Geometry: final body of the model. Coordinates: model frame, mm. A direction names the side the tool comes from. Round coordinates to 2 decimals unless told otherwise and drop trailing zeros. Loops run counter-clockwise (first coordinate to the right, second up) from the corner with the lowest first, then second, coordinate; pieces in that order, holes last. Notation, with made-up numbers: (-14, 38) - (32, 38) arc R5 ccw to (32, 47) - close; hole circle Ø3 at (10, 19.5). An arc over 180 degrees is marked (long way). Answer in a Markdown table with one row per item. Add a question column.
from build123d import *

# Parameters (mm, degrees)
CUT_EXTRUDE1_DEPTH      = 74.786855198
CUT_EXTRUDE1_DEPTH_BACK = 74.786855198
SKETCH3_W               = 2
SKETCH3_H               = 17
CUT_EXTRUDE2_DEPTH      = 44
CIRPATTERN1_COUNT       = 3


with BuildPart() as part:
    # Sketch1 → Revolve1 (revolve)
    with BuildSketch(Plane.XY, mode=Mode.PRIVATE) as revolve1_sk:
        Polygon((8, 0), (11.5, 0), (11.5, 19), (10, 19), (10, 46), (12.5, 46), (16.5, 70), (8, 70), align=None)
    revolve(revolve1_sk.sketch.rotate(Axis((0, 72.635796235, 0), (0, -1, 0)), 90), axis=Axis((0, 72.635796235, 0), (0, -1, 0)))

    # Sketch2 → Cut-Extrude1 (cut, two sides: drawn at the far end of the back side and taken through both)
    with BuildSketch(Plane.XY.offset(-CUT_EXTRUDE1_DEPTH_BACK)):
        with BuildLine():
            Line((2.5, 13), (2.5, 6))
            ThreePointArc((2.5, 6), (0, 3.5), (-2.5, 6))
            Line((-2.5, 6), (-2.5, 13))
            ThreePointArc((-2.5, 13), (0, 15.5), (2.5, 13))
        make_face()
    extrude(amount=CUT_EXTRUDE1_DEPTH + CUT_EXTRUDE1_DEPTH_BACK, mode=Mode.SUBTRACT)

    # Sketch3 → Cut-Extrude2 (cut)
    with BuildSketch(Plane(origin=(0, 70, 0), x_dir=(1, 0, 0), z_dir=(0, 1, 0))):
        with Locations((0, 13.67175851)):
            Rectangle(SKETCH3_W, SKETCH3_H)
    cut_extrude2 = extrude(amount=-CUT_EXTRUDE2_DEPTH, mode=Mode.SUBTRACT)

    # CirPattern1: Cut-Extrude2 ×3 about axis
    cirpattern1_axis = Axis((0, 0, 0), (0, 1, 0))
    for i in range(1, CIRPATTERN1_COUNT):
        add(cut_extrude2.rotate(cirpattern1_axis, i * 360 / CIRPATTERN1_COUNT), mode=Mode.SUBTRACT)


solid = part.part
1) Contact query for flat-ended pins moving along their axis: pin 1 Ø1.8 at (y, z) = (10.5, 10) entering from -X; pin 2 Ø1.1 at (y, z) = (9, 8.5) entering from +X; pin 3 Ø2 at (x, y) = (9, 41.5) entering from +Z. Output: stop coordinate, or through.
2) Section A-A, the plane z = 0. Return the cut outline in (x, y), and give its area (3 significant figures).
3) Pull-direction query (Y, two-part tool) for faces 1 (the flat face through (-10.196, 53.197, 4.732)), 2 (the cylindrical face through (0.1, 3.5, 9.5)), 3 (the flat face through (-9, 70, -5)); classes: pulls with the +Y half, pulls with the -Y half, needs draft (parallel to the pull), parting line crosses it, or undercut.
4) Section C-C, the plane y = 5. Return the cut outline in (x, z).
5) Material intervals for line 1 along X through (y, z) = (14, -2.5); line 2 along Y through (x, z) = (-10, 3); line 3 along X through (y, z) = (18, 0), sorted ascending. Write a range as from..to.
6) Section B-B, the plane y = 54. Return the cut outline in (x, z).
7) Section D-D, the plane y = 29.5. Return the cut outline in (x, z).
8) Reachability of faces 4 (the flat face through (0, 46, 11)), 5 (the flat face through (2.5, 10, -9)), 6 (the flat face through (9.196, 53.197, 6.464)), 7 (the flat face through (1, 53, -11)) from +Z, -Z, +X, -X, +Y, -Y: full face, straight path, thin tool, end or side. Return the list, or none.
Evaluation:
| question | item | result |
|---|---|---|
| 1 | pin 1 | stops at x = -7.03 |
| 1 | pin 2 | stops at x = 8.31 |
| 1 | pin 3 | stops at z = 6 |
| 2 | outline | (-16.5, 70) - (-12.5, 46) - (-10, 46) - (-10, 19) - (-11.5, 19) - (-11.5, 0) - (-8, 0) - (-8, 70) - close; (8, 0) - (11.5, 0) - (11.5, 19) - (10, 19) - (10, 46) - (12.5, 46) - (16.5, 70) - (8, 70) - close |
| 2 | area | 553 mm² |
| 3 | face 1 | needs draft |
| 3 | face 2 | undercut |
| 3 | face 3 | pulls with the +Y half |
| 4 | outline | (-2.29, -11.27) - (-2.29, -7.66) arc R8 cw to (-2.29, 7.66) - (-2.29, 11.27) arc R11.5 ccw to start; (2.29, -11.27) arc R11.5 ccw to (2.29, 11.27) - (2.29, 7.66) arc R8 cw to (2.29, -7.66) - close |
| 5 | line 1 | x = -11.22..-7.6, 7.6..11.22 |
| 5 | line 2 | y = 0..19, 46..70 |
| 5 | line 3 | x = -11.5..-8, 8..11.5 |
| 6 | outline | (-12.45, 6.03) arc R13.83 ccw to (-1, -13.8) - (-1, -7.94) arc R8 cw to (-7.37, 3.1) - close; (-11.45, 7.76) - (-6.37, 4.83) arc R8 cw to (6.37, 4.83) - (11.45, 7.76) arc R13.83 ccw to start; (1, -13.8) arc R13.83 ccw to (12.45, 6.03) - (7.37, 3.1) arc R8 cw to (1, -7.94) - close |
| 7 | outline | (-9.12, 4.11) arc R10 ccw to (-1, -9.95) - (-1, -7.94) arc R8 cw to (-7.37, 3.1) - close; (-8.12, 5.84) - (-6.37, 4.83) arc R8 cw to (6.37, 4.83) - (8.12, 5.84) arc R10 ccw to start; (1, -9.95) arc R10 ccw to (9.12, 4.11) - (7.37, 3.1) arc R8 cw to (1, -7.94) - close |
| 8 | face 4 | +Z |
| 8 | face 5 | +Z, -Z |
| 8 | face 6 | +Y |
| 8 | face 7 | -Z, +Y |
